Job drawing, mm, ordinate dimensions from the low corner. One solid piece. Give positions to 0.01 mm unless a question says otherwise; leave off trailing zeros. Write each loop counter-clockwise with the first axis right and the second up, starting at its lowest first coordinate (ties: lowest second). Pieces come first, ordered by that corner, then holes. Notation, with made-up numbers: (81.5, 63) - (116.5, 63) arc R18 ccw to (116.5, 92) - close; hole circle Ø3 at (58, -22.75). An arc over 180 degrees is marked (long way). Put each result on its own line as item: value. Start each with the question number.
1. Wall check: line 1 (X direction, y = 1.75, z = 6) (3 decimals); line 2 (X direction, y = 1.15, z = 13.25) (3 decimals). Give the ranges that are in metal, low to high.
2. Cut at A-A on z = 2.75. List the corners of the cut face in (x, y), and give its area (3 significant figures).
3. Cut at B-B on y = 1.1. List the corners of the cut face in (x, z), and give its area (3 significant figures).
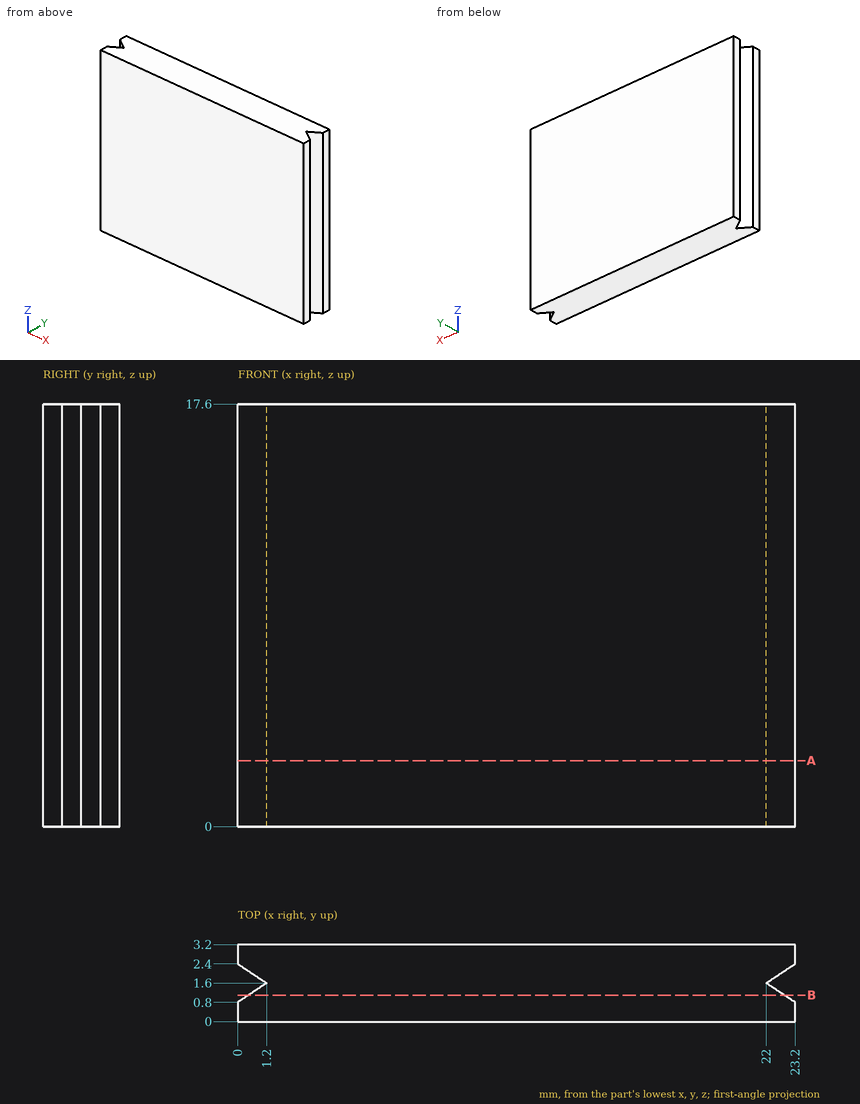
Report:
1. line 1: x = 0.975 to 22.225
1. line 2: x = 0.525 to 22.675
2. outline: (0, 0) - (23.2, 0) - (23.2, 0.8) - (22, 1.6) - (23.2, 2.4) - (23.2, 3.2) - (0, 3.2) - (0, 2.4) - (1.2, 1.6) - (0, 0.8) - close
2. area: 72.3 mm²
3. outline: (0.45, 0) - (22.75, 0) - (22.75, 17.6) - (0.45, 17.6) - close
3. area: 392 mm²
